from build123d import *

# Parameters (mm, degrees)
SKETCH1_R           = 1.5
BOSS_EXTRUDE1_DEPTH = 3


with BuildPart() as part:
    # Sketch1 → Boss-Extrude1 (new body)
    with BuildSketch(Plane.XY):
        with BuildLine():
            Line((-10, 0), (-10, 3))
            ThreePointArc((-10, 3), (-9.622914027, 8.055937104), (-8.5, 13))
            ThreePointArc((-8.5, 13), (-4.008343892, 32.776251584), (-2.5, 53))
            Line((-2.5, 53), (-2.5, 103))
            Line((-2.5, 103), (-9.863636364, 89.5))
            Line((-9.863636364, 89.5), (-16, 89.5))
            Line((-16, 89.5), (-16, 94.5))
            Line((-16, 94.5), (-11, 94.5))
            Line((-11, 94.5), (-5, 105.5))
            Line((-5, 105.5), (-11, 116.5))
            Line((-11, 116.5), (-16, 116.5))
            Line((-16, 116.5), (-16, 121.5))
            Line((-16, 121.5), (-9.863636364, 121.5))
            Line((-9.863636364, 121.5), (-2.5, 108))
            Line((-2.5, 108), (2.5, 108))
            Line((2.5, 108), (9.863636364, 121.5))
            Line((9.863636364, 121.5), (16, 121.5))
            Line((16, 121.5), (16, 116.5))
            Line((16, 116.5), (11, 116.5))
            Line((11, 116.5), (5, 105.5))
            Line((5, 105.5), (11, 94.5))
            Line((11, 94.5), (16, 94.5))
            Line((16, 94.5), (16, 89.5))
            Line((16, 89.5), (9.863636364, 89.5))
            Line((9.863636364, 89.5), (2.5, 103))
            Line((2.5, 103), (2.5, 53))
            ThreePointArc((2.5, 53), (4.008343892, 32.776251584), (8.5, 13))
            ThreePointArc((8.5, 13), (9.622914027, 8.055937104), (10, 3))
            Line((10, 3), (10, 0))
            Line((10, 0), (6, 0))
            Line((6, 0), (6, 3))
            Line((6, 3), (2, 3))
            Line((2, 3), (2, 0))
            Line((2, 0), (-2, 0))
            Line((-2, 0), (-2, 3))
            Line((-2, 3), (-6, 3))
            Line((-6, 3), (-6, 0))
            Line((-6, 0), (-10, 0))
        make_face()
        with Locations((-13.5, 92)):
            Circle(SKETCH1_R, mode=Mode.SUBTRACT)
        with Locations(Location((13.5, 92, 0), (0, 0, 180))):
            Circle(SKETCH1_R, mode=Mode.SUBTRACT)
        with Locations((13.5, 119)):
            Circle(SKETCH1_R, mode=Mode.SUBTRACT)
        with Locations(Location((-13.5, 119, 0), (0, 0, 180))):
            Circle(SKETCH1_R, mode=Mode.SUBTRACT)
    extrude(amount=BOSS_EXTRUDE1_DEPTH)


solid = part.part
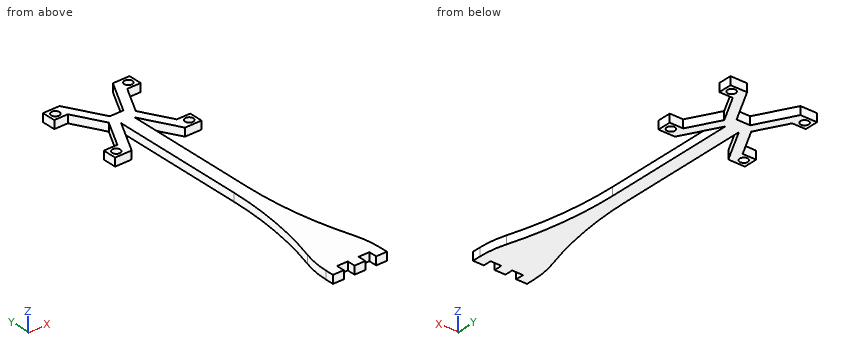
Can you work these out from the model? Positions are in its coordinate system, mm. Coordinates: 2 decimals unless noted, no trailing zeros. Loops run counter-clockwise (first coordinate to the right, second up) from the corner with the lowest first, then second, coordinate; pieces in that order, holes last. Notation, with made-up numbers: (57, 55.5) - (96, 55.5) arc R30 cw to (96, 85.5) - close; hole circle Ø6 at (29, 56). An arc over 180 degrees is marked (long way). Answer as a JSON object with one key per item and string values. Group by question number.
Item 1: If we section it at D-D (x = 0): List the corners of the cut face in (y, z) for me, plus the area to 3 significant figures.
Item 2: If I drill on L1, parallel to Y at x = -13.5, z = 1.9; L2, parallel to X at y = 92, z = 1.15; L3, parallel to X at y = 119, z = 2.15, over which ranges is the centre line in solid material (lowest first)? Write a range as from..to.
Item 3: If we section it at C-C (z = 1.9): State how many separate pieces and enclosed holes the cut face has, plus the area to 3 significant figures.
Item 4: For pin 1 (4 mm diameter, centred on x = -13.5, y = 92, fed in from -Z); pin 2 (1.5 mm diameter, centred on x = 12, z = 1, fed in from -Y); pin 3 (0.9 mm diameter, centred on y = 68, z = 1, fed in from +X), each with a flat end and sliding along its axis, tell me the tip position at first contact or that it passes through.
Item 5: If we section it at A-A (y = 92): List the corners of the cut face in (x, z) for me, plus the area to 3 significant figures.
Item 6: If we section it at B-B (x = -13.5): List the corners of the cut face in (y, z) for me.
Returned:
{
 "1": {"outline": "(0, 0) - (108, 0) - (108, 3) - (0, 3) - close", "area": "324 mm²"},
 "2": {"L1": "y = 89.5..90.5, 93.5..94.5, 116.5..117.5, 120.5..121.5", "L2": "x = -16..-15, -12..-8.5, -2.5..2.5, 8.5..12, 15..16", "L3": "x = -16..-15, -12..-8.5, 8.5..12, 15..16"},
 "3": {"separate pieces": "1", "enclosed holes": "4", "area": "1,140 mm²"},
 "4": {"pin 1": "stops at z = 0", "pin 2": "stops at y = 89.5", "pin 3": "stops at x = 2.5"},
 "5": {"outline": "(-16, 0) - (-15, 0) - (-15, 3) - (-16, 3) - close; (-12, 0) - (-8.5, 0) - (-8.5, 3) - (-12, 3) - close; (-2.5, 0) - (2.5, 0) - (2.5, 3) - (-2.5, 3) - close; (8.5, 0) - (12, 0) - (12, 3) - (8.5, 3) - close; (15, 0) - (16, 0) - (16, 3) - (15, 3) - close", "area": "42.0 mm²"},
 "6": {"outline": "(89.5, 0) - (90.5, 0) - (90.5, 3) - (89.5, 3) - close; (93.5, 0) - (94.5, 0) - (94.5, 3) - (93.5, 3) - close; (116.5, 0) - (117.5, 0) - (117.5, 3) - (116.5, 3) - close; (120.5, 0) - (121.5, 0) - (121.5, 3) - (120.5, 3) - close"}
}
